Design review of the part built by this model. Coordinates are the model's own, in mm. A direction names the side the tool comes from. Give positions to 0.01 mm unless a question says otherwise; leave off trailing zeros. Loops run counter-clockwise (first coordinate to the right, second up) from the corner with the lowest first, then second, coordinate; pieces in that order, holes last. Notation, with made-up numbers: M -27.5,20 L 8.5,20 A18 cw 8.5,55 Z; hole C 18.5,60.5 d9. An arc over 180 degrees is marked long. Use one line per item in the form item = value. Start each with the question number.
from build123d import *

# Parameters (mm, degrees)
SKETCH3_R           = 10
BOSS_EXTRUDE1_DEPTH = 18
SKETCH4_W           = 2.5
SKETCH4_H           = 8
BOSS_EXTRUDE2_DEPTH = 25
CUT_EXTRUDE1_REACH  = 33.579
SKETCH5_R           = 2.6
SKETCH7_W           = 17
SKETCH7_H           = 7
CUT_EXTRUDE3_DEPTH  = 6
SKETCH8_W           = 2
SKETCH8_H           = 7
CUT_EXTRUDE4_DEPTH  = 4
SKETCH11_W          = 5.5
SKETCH11_H          = 21
CUT_EXTRUDE7_DEPTH  = 1.5
CUT_EXTRUDE5_DEPTH  = 43
BOSS_EXTRUDE3_DEPTH = 1.5


with BuildPart() as part:
    # Sketch3 → Boss-Extrude1 (new body)
    with BuildSketch(Plane(origin=(0, 0, 0), x_dir=(1, 0, 0), z_dir=(0, 1, 0))):
        with Locations(Location((0, 0, 0), (0, 0, 270))):
            Circle(SKETCH3_R)
    extrude(amount=BOSS_EXTRUDE1_DEPTH)

    # Sketch4 → Boss-Extrude2 (add)
    with BuildSketch(Plane(origin=(0, 0, 0), x_dir=(-1, 0, 0), z_dir=(0, -1, 0))):
        with Locations((7.75, 0)):
            Rectangle(SKETCH4_W, SKETCH4_H)
    extrude(amount=BOSS_EXTRUDE2_DEPTH)

    # Sketch5 → Cut-Extrude1 (cut, up to next)
    with BuildSketch(Plane(origin=(-6.5, 0, 0), x_dir=(0, 0, -1), z_dir=(1, 0, 0)), mode=Mode.PRIVATE) as cut_extrude1_sk1:
        with Locations((0, -13.4)):
            Circle(SKETCH5_R)
    cut_extrude1_tool1 = extrude(cut_extrude1_sk1.sketch, amount=-CUT_EXTRUDE1_REACH, mode=Mode.PRIVATE) & part.part
    add(cut_extrude1_tool1.solids().sort_by_distance((-6.5, -13.4, 0))[0], mode=Mode.SUBTRACT)

    # Sketch7 → Cut-Extrude3 (cut)
    with BuildSketch(Plane(origin=(0, 18, 0), x_dir=(1, 0, 0), z_dir=(0, 1, 0))):
        Rectangle(SKETCH7_W, SKETCH7_H)
    extrude(amount=-CUT_EXTRUDE3_DEPTH, mode=Mode.SUBTRACT)

    # Sketch8 → Cut-Extrude4 (cut)
    with BuildSketch(Plane(origin=(0, 12, 0), x_dir=(1, 0, 0), z_dir=(0, 1, 0))):
        with Locations((-2.25, 0)):
            Rectangle(SKETCH8_W, SKETCH8_H)
    extrude(amount=-CUT_EXTRUDE4_DEPTH, mode=Mode.SUBTRACT)

    # Sketch11 → Cut-Extrude7 (cut)
    with BuildSketch(Plane.ZY.offset(9)):
        with Locations((0, -13.4)):
            Rectangle(SKETCH11_W, SKETCH11_H)
    extrude(amount=-CUT_EXTRUDE7_DEPTH, mode=Mode.SUBTRACT)

    # Sketch9 → Cut-Extrude5 (cut)
    with BuildSketch(Plane.XZ):
        with BuildLine():
            Line((8.351646544, -5.5), (-8.351646544, -5.5))
            ThreePointArc((-8.351646544, -5.5), (0, -10), (8.351646544, -5.5))
        make_face()
        with BuildLine():
            Line((8.351646544, 5.5), (-8.351646544, 5.5))
            ThreePointArc((-8.351646544, 5.5), (0, 10), (8.351646544, 5.5))
        make_face()
    extrude(amount=-CUT_EXTRUDE5_DEPTH, mode=Mode.SUBTRACT)

    # Sketch10 → Boss-Extrude3 (add)
    with BuildSketch(Plane.ZY.offset(9)):
        Polygon((-2.749970665, -23.9), (-2.749970665, -16.8), (-1.499970665, -23.9), align=None)
        Polygon((1.499970665, -23.9), (2.749970665, -23.9), (2.749970665, -16.8), align=None)
        Polygon((2.749970665, -2.9), (2.749970665, -10), (1.499970665, -2.9), align=None)
        Polygon((-1.499970665, -2.9), (-2.749970665, -2.9), (-2.749970665, -10), align=None)
    extrude(amount=-BOSS_EXTRUDE3_DEPTH)


solid = part.part
Q1. Take a section at A-A on y = 11.5. Give the boundary of the cut face in (x, z), plus the area to 3 significant figures.
Q2. Take a section at B-B on z = 0. Give the boundary of the cut face in (x, y), plus the area to 3 significant figures.
Q3. For faces 5 (the flat face through (-8, -14, 2.75)), 6 (the flat face through (-1.25, 10, 0)), 7 (the flat face through (0, 9, 5.5)), 8 (the flat face through (-8, -2.9, 0)), 9 (the flat face through (-9, -10, 3)), list the 3-axis set-ups (+Z, -Z, +X, -X, +Y, -Y) from which the entire face can be reached by the end or side of a thin tool; tool diameter is ignored.
Q4. The part is to be moulded in two halves that separate along Y. For faces 1 (the flat face through (-8.26, -20.3, -2.134)), 2 (the flat face through (-8, -12, -4)), 3 (the flat face through (-8, -25, 0)), 4 (the flat face through (-8.26, -20.3, 2.134)), say which applies: pulls with the +Y half, pulls with the -Y half, needs draft (parallel to the pull), parting line crosses it, or undercut.
Q5. Take a section at C-C on x = -6. Give the boundary of the cut face in (y, z).
Q6. Take a section at D-D on y = -13.4. Give the boundary of the cut face in (x, z), plus the area to 3 significant figures.
Q7. Clearance check with flat-ended pins moving along their axes: pin 1 Ø1 at (y, z) = (-12, -3.5) entering from +X; pin 2 Ø1.6 at (x, y) = (-8.5, -7.5) entering from -Z; pin 3 Ø4 at (y, z) = (-13.5, 2.5) entering from -X. State where each tip first meets the part, or that it passes through.
Q8. Wall thickness on probe 1 along Z at (x, y) = (-3, 14); probe 2 along Y at (x, z) = (-6.85, 0); probe 3 along X at (y, z) = (-13, 3.5): over which ranges is each line inside the solid? List them lowest first.
Response values:
q1.outline = M -8.35,-5.5 L 8.35,-5.5 A10 ccw 8.35,5.5 L -8.35,5.5 A10 ccw Z; hole M -3.25,-3.5 L -1.25,-3.5 L -1.25,3.5 L -3.25,3.5 Z
q1.area = 194 mm^2
q2.outline = M -10,0 L -9,0 L -9,-2.9 L -7.5,-2.9 L -7.5,-10.8 L -6.5,-10.8 L -6.5,0 L 10,0 L 10,18 L 8.5,18 L 8.5,12 L -1.25,12 L -1.25,8 L -3.25,8 L -3.25,12 L -8.5,12 L -8.5,18 L -10,18 Z; M -9,-25 L -6.5,-25 L -6.5,-16 L -7.5,-16 L -7.5,-23.9 L -9,-23.9 Z
q2.area = 276 mm^2
q3.face_5 = none
q3.face_6 = +Y
q3.face_7 = +Z, +X, -X, +Y, -Y
q3.face_8 = -X
q3.face_9 = +Z, -Z, -X, -Y
q4.face_1 = undercut
q4.face_2 = needs draft
q4.face_3 = pulls with the -Y half
q4.face_4 = undercut
q5.outline = M 0,-5.5 L 18,-5.5 L 18,-3.5 L 12,-3.5 L 12,3.5 L 18,3.5 L 18,5.5 L 0,5.5 Z
q6.outline = M -9,-4 L -6.5,-4 L -6.5,-2.6 L -7.5,-2.6 L -7.5,-2.75 L -9,-2.75 Z; M -9,2.75 L -7.5,2.75 L -7.5,2.6 L -6.5,2.6 L -6.5,4 L -9,4 Z
q6.area = 6.55 mm^2
q7.pin_1 = -6.5
q7.pin_2 = -4
q7.pin_3 = -9
q8.probe_1 = -5.5 to -3.5, 3.5 to 5.5
q8.probe_2 = -25 to -16, -10.8 to 12
q8.probe_3 = -9 to -6.5
